Can you work these out from the drawing? Everything is in mm from the part's minimum corner. Round coordinates to 2 decimals unless told otherwise and drop trailing zeros. Loops run counter-clockwise (first coordinate to the right, second up) from the corner with the lowest first, then second, coordinate; pieces in that order, holes last. Notation, with made-up numbers: M 83.5,-38 L 132.5,-38 A19 cw 132.5,-23 Z; hole C 54.25,-37.5 d7. An arc over 180 degrees is marked long. One line per question, with ' | ' between items. Start each with the question number.
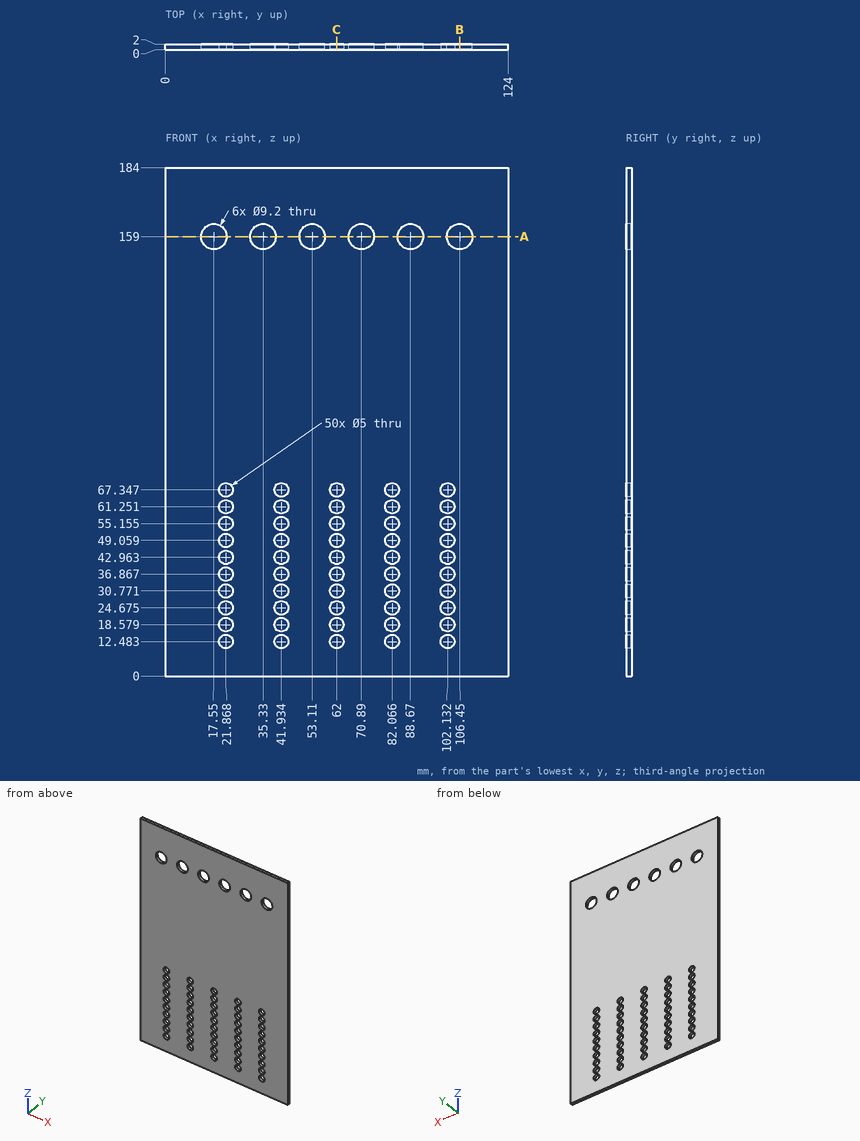
1) Imagine slicing it at A-A (z = 159). Write out the boundary of the cut face in (x, y), then the cut area to 3 significant figures.
2) Please list where these lines run through material, in increasing order: L1, parallel to X at y = 0.15, z = 12 (1 decimal); L2, parallel to X at y = 1.55, z = 44.5 (1 decimal); L3, parallel to Z at x = 106.5, y = 0.2. Write a range as from..to.
3) Imagine slicing it at B-B (x = 106.45). Write out the boundary of the cut face in (y, z).
4) Imagine slicing it at C-C (x = 62). State how many separate pieces and enclosed holes the cut face has, then the cut area to 3 significant figures.
5) I'm going to push a flat-ended pin straight in: pin 1 Ø3 at (x, z) = (62, 49.06) entering from +Y. Where does the tip first touch, or does it pass through?
Results are:
1) outline: M 0,0 L 12.95,0 L 12.95,2 L 0,2 Z; M 22.15,0 L 30.73,0 L 30.73,2 L 22.15,2 Z; M 39.93,0 L 48.51,0 L 48.51,2 L 39.93,2 Z; M 57.71,0 L 66.29,0 L 66.29,2 L 57.71,2 Z; M 75.49,0 L 84.07,0 L 84.07,2 L 75.49,2 Z; M 93.27,0 L 101.85,0 L 101.85,2 L 93.27,2 Z; M 111.05,0 L 124,0 L 124,2 L 111.05,2 Z | area: 138 mm²
2) L1: 0..19.4, 24.3..39.5, 44.4..59.5, 64.5..79.6, 84.5..99.7, 104.6..124 | L2: 0..19.9, 23.8..40, 43.9..60, 64..80.1, 84..100.2, 104.1..124 | L3: 0..154.4, 163.6..184
3) outline: M 0,0 L 2,0 L 2,154.4 L 0,154.4 Z; M 0,163.6 L 2,163.6 L 2,184 L 0,184 Z
4) separate pieces: 11 | enclosed holes: 0 | area: 268 mm²
5) pin 1: through
